Check sheet for the modelled part. Datum: model origin and axes. Units: mm. Face numbers are marked on the shaded views. Coordinates: 2 decimals unless noted, no trailing zeros. Loops run counter-clockwise (first coordinate to the right, second up) from the corner with the lowest first, then second, coordinate; pieces in that order, holes last. Notation, with made-up numbers: M 47.25,60.5 L 60.25,60.5 A17 cw 60.25,87.5 Z; hole C 74,-1.75 d9. An arc over 180 degrees is marked long. Return JSON: item names as keys, results as strings.
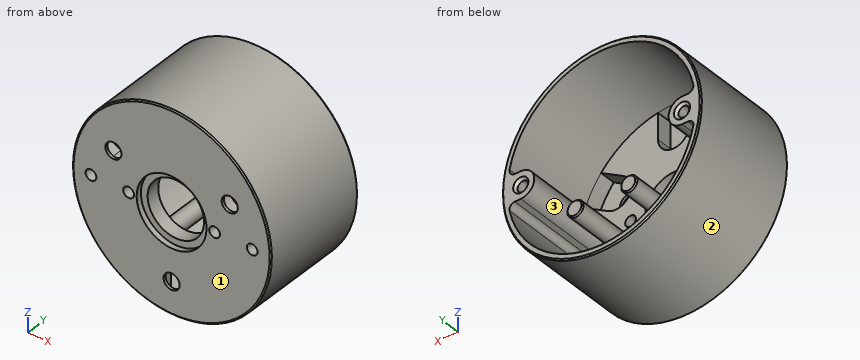
from build123d import *
from OCP.BRepFilletAPI import BRepFilletAPI_MakeChamfer

# Parameters (mm, degrees)
SKETCH1_R            = 18.5
BOSS_EXTRUDE1_DEPTH  = 20.5
SKETCH2_R            = 17.5
CUT_EXTRUDE1_DEPTH   = 17
CUT_EXTRUDE2_REACH   = 35.238
SKETCH4_R            = 5.25
BOSS_EXTRUDE2_START  = 17
SKETCH5_R            = 2.5
BOSS_EXTRUDE2_DEPTH  = 17
FILLET1_R            = 1
SKETCH6_R            = 1
CUT_EXTRUDE3_DEPTH   = 34.237779709
FILLET1_OF_MIRROR1_R = 1
SKETCH7_R            = 2.9
CUT_EXTRUDE4_DEPTH   = 3
CIRPATTERN1_COUNT    = 6
SKETCH8_R            = 6.5
CUT_EXTRUDE5_DEPTH   = 1
CUT_EXTRUDE6_REACH   = 35.238
SKETCH9_R            = 1
CUT_EXTRUDE7_REACH   = 34.932
SKETCH11_R           = 1.5
CIRPATTERN2_COUNT    = 3
SKETCH12_R           = 1.5
BOSS_EXTRUDE3_DEPTH  = 17
CHAMFER1_SIZE        = 0.5
CHAMFER1_SIZE2       = 0.419549816
CHAMFER2_SIZE        = 0.25
CHAMFER2_SIZE2       = 0.209774908
CHAMFER3_SIZE        = 0.25
CHAMFER3_SIZE2       = 0.209774908


with BuildPart() as part:
    # Sketch1 → Boss-Extrude1 (new body)
    with BuildSketch(Plane(origin=(0, 0, 0), x_dir=(1, 0, 0), z_dir=(0, 1, 0))):
        with Locations(Location((0, 0, 0), (0, 0, 270))):
            Circle(SKETCH1_R)
    extrude(amount=BOSS_EXTRUDE1_DEPTH)

    # Sketch2 → Cut-Extrude1 (cut)
    with BuildSketch(Plane(origin=(0, 20.5, 0), x_dir=(1, 0, 0), z_dir=(0, 1, 0))):
        with Locations(Location((0, 0, 0), (0, 0, 270))):
            Circle(SKETCH2_R)
    extrude(amount=-CUT_EXTRUDE1_DEPTH, mode=Mode.SUBTRACT)

    # Sketch4 → Cut-Extrude2 (cut, up to next)
    with BuildSketch(Plane.XZ, mode=Mode.PRIVATE) as cut_extrude2_sk1:
        with Locations(Location((0, 0, 0), (0, 0, 270))):
            Circle(SKETCH4_R)
    cut_extrude2_tool1 = extrude(cut_extrude2_sk1.sketch, amount=-CUT_EXTRUDE2_REACH, mode=Mode.PRIVATE) & part.part
    add(cut_extrude2_tool1.solids().sort_by_distance((0, 0, 0))[0], mode=Mode.SUBTRACT)

    # Sketch5 → Boss-Extrude2 (add)
    with BuildSketch(Plane(origin=(0, 3.5, 0), x_dir=(1, 0, 0), z_dir=(0, 1, 0)).offset(BOSS_EXTRUDE2_START)):
        with Locations((-15, 0)):
            Circle(SKETCH5_R)
        with BuildLine():
            ThreePointArc((-17.5, 0), (-16.767766953, 1.767766953), (-15, 2.5))
            Line((-15, 2.5), (-17.320508076, 2.5))
            ThreePointArc((-17.320508076, 2.5), (-17.45506934, 1.253217594), (-17.5, 0))
        make_face()
        with BuildLine():
            ThreePointArc((-15, -2.5), (-16.767766953, -1.767766953), (-17.5, 0))
            ThreePointArc((-17.5, 0), (-17.45506934, -1.253217594), (-17.320508076, -2.5))
            Line((-17.320508076, -2.5), (-15, -2.5))
        make_face()
    boss_extrude2 = extrude(amount=-BOSS_EXTRUDE2_DEPTH)

    # Fillet1
    fillet1_edges = [part.edges().sort_by_distance(p)[0] for p in [
        (-17.320508076, 12, -2.5),
        (-17.320508076, 12, 2.5),
    ]]
    fillet(fillet1_edges, radius=FILLET1_R)

    # Sketch6 → Cut-Extrude3 (cut, through all)
    with BuildSketch(Plane(origin=(0, 20.5, 0), x_dir=(1, 0, 0), z_dir=(0, 1, 0))):
        with Locations(Location((-15, 0, 0), (0, 0, 270))):
            Circle(SKETCH6_R)
    cut_extrude3 = extrude(amount=-CUT_EXTRUDE3_DEPTH, mode=Mode.SUBTRACT)

    # Mirror1: Boss-Extrude2, Cut-Extrude3 across plane
    add(boss_extrude2.mirror(Plane(origin=(0, 0, 0), x_dir=(0, 0, 1), z_dir=(1, 0, 0))))
    add(cut_extrude3.mirror(Plane(origin=(0, 0, 0), x_dir=(0, 0, 1), z_dir=(1, 0, 0))), mode=Mode.SUBTRACT)

    # Fillet1 of Mirror1
    fillet1_of_mirror1_edges = [part.edges().sort_by_distance(p)[0] for p in [
        (17.320508076, 12, -2.5),
        (17.320508076, 12, 2.5),
    ]]
    fillet(fillet1_of_mirror1_edges, radius=FILLET1_OF_MIRROR1_R)

    # Sketch7 → Cut-Extrude4 (cut)
    with BuildSketch(Plane(origin=(0, 3.5, 0), x_dir=(1, 0, 0), z_dir=(0, 1, 0))):
        with Locations((0, 12.4)):
            Circle(SKETCH7_R)
        with BuildLine():
            Line((-2.9, 17.258041604), (-2.9, 12.4))
            ThreePointArc((-2.9, 12.4), (0, 15.3), (2.9, 12.4))
            Line((2.9, 12.4), (2.9, 17.258041604))
            ThreePointArc((2.9, 17.258041604), (0, 17.5), (-2.9, 17.258041604))
        make_face()
    cut_extrude4 = extrude(amount=-CUT_EXTRUDE4_DEPTH, mode=Mode.SUBTRACT)

    # CirPattern1: Cut-Extrude4 ×6 about axis
    cirpattern1_axis = Axis((0, 0, 0), (0, 1, 0))
    for i in range(1, CIRPATTERN1_COUNT):
        add(cut_extrude4.rotate(cirpattern1_axis, i * 360 / CIRPATTERN1_COUNT), mode=Mode.SUBTRACT)

    # Sketch8 → Cut-Extrude5 (cut)
    with BuildSketch(Plane.XZ):
        with Locations(Location((0, 0, 0), (0, 0, 270))):
            Circle(SKETCH8_R)
    extrude(amount=-CUT_EXTRUDE5_DEPTH, mode=Mode.SUBTRACT)

    # Sketch9 → Cut-Extrude6 (cut, up to next)
    with BuildSketch(Plane.XZ, mode=Mode.PRIVATE) as cut_extrude6_sk1:
        with Locations(Location((-8, 0, 0), (0, 0, 270))):
            Circle(SKETCH9_R)
    cut_extrude6_tool1 = extrude(cut_extrude6_sk1.sketch, amount=-CUT_EXTRUDE6_REACH, mode=Mode.PRIVATE) & part.part
    # Sketch9 → Cut-Extrude6 (cut, up to next)
    with BuildSketch(Plane.XZ, mode=Mode.PRIVATE) as cut_extrude6_sk2:
        with Locations(Location((8, 0, 0), (0, 0, 270))):
            Circle(SKETCH9_R)
    cut_extrude6_tool2 = extrude(cut_extrude6_sk2.sketch, amount=-CUT_EXTRUDE6_REACH, mode=Mode.PRIVATE) & part.part
    add(cut_extrude6_tool1.solids().sort_by_distance((-8, 0, 0))[0], mode=Mode.SUBTRACT)
    add(cut_extrude6_tool2.solids().sort_by_distance((8, 0, 0))[0], mode=Mode.SUBTRACT)

    # Sketch11 → Cut-Extrude7 (cut, up to next)
    with BuildSketch(Plane(origin=(0, 0.5, 0), x_dir=(1, 0, 0), z_dir=(0, 1, 0)), mode=Mode.PRIVATE) as cut_extrude7_sk1:
        with Locations(Location((0, 12.5, 0), (0, 0, 270))):
            Circle(SKETCH11_R)
    cut_extrude7_tool1 = extrude(cut_extrude7_sk1.sketch, amount=-CUT_EXTRUDE7_REACH, mode=Mode.PRIVATE) & part.part
    cut_extrude7 = cut_extrude7_tool1.solids().sort_by_distance((0, 0.5, -12.5))[0]
    add(cut_extrude7, mode=Mode.SUBTRACT)

    # CirPattern2: Cut-Extrude7 ×3 about axis
    cirpattern2_axis = Axis((0, 0, 0), (0, 1, 0))
    for i in range(1, CIRPATTERN2_COUNT):
        add(cut_extrude7.rotate(cirpattern2_axis, i * 360 / CIRPATTERN2_COUNT), mode=Mode.SUBTRACT)

    # Sketch12 → Boss-Extrude3 (add)
    with BuildSketch(Plane(origin=(0, 3.5, 0), x_dir=(1, 0, 0), z_dir=(0, 1, 0))):
        with Locations(Location((-5, 8.660254038, 0), (0, 0, 270))):
            Circle(SKETCH12_R)
        with Locations(Location((5, 8.660254038, 0), (0, 0, 270))):
            Circle(SKETCH12_R)
    extrude(amount=BOSS_EXTRUDE3_DEPTH)

    # Chamfer1: one chamfer whose edges measure the first distance from different faces: ONE call of the kernel's chamfer builder (chamfer() names one face for all edges)
    chamfer1_edges_1 = [part.edges().sort_by_distance(p)[0] for p in [
        (-15, 20.5, -1),
    ]]
    chamfer1_side_1 = [part.faces().sort_by_distance(p)[0] for p in [
        (0, 20.5, -18.023259018),
    ]]
    chamfer1_edges_2 = [part.edges().sort_by_distance(p)[0] for p in [
        (15, 20.5, -1),
    ]]
    chamfer1_side_2 = [part.faces().sort_by_distance(p)[0] for p in [
        (15, 10.25, -1),
    ]]
    chamfer1 = BRepFilletAPI_MakeChamfer(part.part.solid().wrapped)
    for e in chamfer1_edges_1:
        chamfer1.Add(CHAMFER1_SIZE, CHAMFER1_SIZE2, e.wrapped, chamfer1_side_1[0].wrapped)  # the first distance lies on this face
    for e in chamfer1_edges_2:
        chamfer1.Add(CHAMFER1_SIZE, CHAMFER1_SIZE2, e.wrapped, chamfer1_side_2[0].wrapped)  # the first distance lies on this face
    add(Compound.cast(chamfer1.Shape()), mode=Mode.REPLACE)

    # Chamfer2: one chamfer whose edges measure the first distance from different faces: ONE call of the kernel's chamfer builder (chamfer() names one face for all edges)
    chamfer2_edges_1 = [part.edges().sort_by_distance(p)[0] for p in [
        (-5, 20.5, -10.160254038),
    ]]
    chamfer2_side_1 = [part.faces().sort_by_distance(p)[0] for p in [
        (-5, 12, -10.160254038),
    ]]
    chamfer2_edges_2 = [part.edges().sort_by_distance(p)[0] for p in [
        (5, 20.5, -10.160254038),
    ]]
    chamfer2_side_2 = [part.faces().sort_by_distance(p)[0] for p in [
        (5, 12, -10.160254038),
    ]]
    chamfer2 = BRepFilletAPI_MakeChamfer(part.part.solid().wrapped)
    for e in chamfer2_edges_1:
        chamfer2.Add(CHAMFER2_SIZE, CHAMFER2_SIZE2, e.wrapped, chamfer2_side_1[0].wrapped)  # the first distance lies on this face
    for e in chamfer2_edges_2:
        chamfer2.Add(CHAMFER2_SIZE, CHAMFER2_SIZE2, e.wrapped, chamfer2_side_2[0].wrapped)  # the first distance lies on this face
    add(Compound.cast(chamfer2.Shape()), mode=Mode.REPLACE)

    # Chamfer3: one chamfer whose edges measure the first distance from different faces: ONE call of the kernel's chamfer builder (chamfer() names one face for all edges)
    chamfer3_edges_1 = [part.edges().sort_by_distance(p)[0] for p in [
        (0, 0, -18.5),
    ]]
    chamfer3_side_1 = [part.faces().sort_by_distance(p)[0] for p in [
        (0, 0, -17.976740982),
    ]]
    chamfer3_edges_2 = [part.edges().sort_by_distance(p)[0] for p in [
        (0, 20.5, -18.5),
    ]]
    chamfer3_side_2 = [part.faces().sort_by_distance(p)[0] for p in [
        (0, 10.25, -18.5),
    ]]
    chamfer3 = BRepFilletAPI_MakeChamfer(part.part.solid().wrapped)
    for e in chamfer3_edges_1:
        chamfer3.Add(CHAMFER3_SIZE, CHAMFER3_SIZE2, e.wrapped, chamfer3_side_1[0].wrapped)  # the first distance lies on this face
    for e in chamfer3_edges_2:
        chamfer3.Add(CHAMFER3_SIZE, CHAMFER3_SIZE2, e.wrapped, chamfer3_side_2[0].wrapped)  # the first distance lies on this face
    add(Compound.cast(chamfer3.Shape()), mode=Mode.REPLACE)


solid = part.part
1) Scan lines: line 1 along X through (y, z) = (2.7, 0); line 2 along X through (y, z) = (11.5, 0); line 3 along Z through (x, y) = (15, 6.5). Record each from-to range of solid material in increasing order. Write a range as [from, to].
Answers:
{"line 1": "[-18.5, -16], [-14, -9], [-7, -5.25], [5.25, 7], [9, 14], [16, 18.5]", "line 2": "[-18.5, -16], [-14, -12.5], [12.5, 14], [16, 18.5]", "line 3": "[-10.83, -9.01], [-2.5, -1], [1, 2.5], [9.01, 10.83]"}
2) Section check B-B on x = 0. Record the cut outline in (y, z), then the cut area to 3 significant figures.
Answers:
{"outline": "M 0,-18.25 L 0.21,-18.5 L 20.25,-18.5 L 20.5,-18.29 L 20.5,-17.5 L 0.5,-17.5 L 0.5,-14 L 0,-14 Z; M 0,-11 L 0.5,-11 L 0.5,-9.5 L 3.5,-9.5 L 3.5,-5.25 L 1,-5.25 L 1,-6.5 L 0,-6.5 Z; M 0,6.5 L 1,6.5 L 1,5.25 L 3.5,5.25 L 3.5,9.5 L 0.5,9.5 L 0.5,17.5 L 20.5,17.5 L 20.5,18.29 L 20.25,18.5 L 0.21,18.5 L 0,18.25 Z", "area": "74.6 mm²"}
3) Draft check along X on the marked faces 1, 2 and 3. Enter one of: +X half, -X half, draft (parallel to the pull), parting line (faces both ways), or undercut.
Answers:
{"face 1": "draft", "face 2": "parting line", "face 3": "undercut"}
4) Go/stop test with flat-tipped pins: pin 1 Ø10 at (y, z) = (8, -1.5) entering from -X; pin 2 Ø1.2 at (x, y) = (15.5, 9.5) entering from -Z; pin 3 Ø2.5 at (x, z) = (15, 0) entering from +Y. Record where each tip stops, or that it passes through.
Answers:
{"pin 1": "x = -18.5", "pin 2": "z = -10.97", "pin 3": "y = 20.3"}
5) Section check C-C on y = 2.5. Count the separate pieces of the cut face and the enclosed holes in it, then the cut area to 3 significant figures.
Answers:
{"separate pieces": "1", "enclosed holes": "11", "area": "722 mm²"}
6) Section check A-A on y = 14.75. Record the cut outline in (x, z), then the cut area to 3 significant figures.
Answers:
{"outline": "C 0,0 d37; C -5,-8.66 d3; C 5,-8.66 d3; hole M -17.1,-3.71 A17.5 ccw 17.1,-3.71 A1 ccw 16.12,-2.5 L 15,-2.5 A2.5 cw 15,2.5 L 16.12,2.5 A1 ccw 17.1,3.71 A17.5 ccw -17.1,3.71 A1 ccw -16.12,2.5 L -15,2.5 A2.5 cw -15,-2.5 L -16.12,-2.5 A1 ccw Z; hole C -15,0 d2; hole C 15,0 d2", "area": "166 mm²"}
